```python
from build123d import *

# Parameters (mm, degrees)
BOSS_EXTRUDE1_DEPTH = 20
SKETCH2_R           = 3.7
CUT_EXTRUDE1_DEPTH  = 20
SKETCH3_R           = 3.7
CUT_EXTRUDE2_DEPTH  = 20


with BuildPart() as part:
    # Sketch1 → Boss-Extrude1 (new body)
    with BuildSketch(Plane.XY):
        Polygon((1.5, -10), (18.5, -10), (18.5, -7), (1.5, -7), (1.5, 10), (-1.5, 10), (-1.5, -10), align=None)
    extrude(amount=BOSS_EXTRUDE1_DEPTH)

    # Sketch2 → Cut-Extrude1 (cut)
    with BuildSketch(Plane(origin=(0, -7, 0), x_dir=(1, 0, 0), z_dir=(0, 1, 0))):
        with Locations(Location((10, -10, 0), (0, 0, 270))):
            Circle(SKETCH2_R)
    extrude(amount=-CUT_EXTRUDE1_DEPTH, mode=Mode.SUBTRACT)

    # Sketch3 → Cut-Extrude2 (cut)
    with BuildSketch(Plane(origin=(1.5, 0, 0), x_dir=(0, 0, -1), z_dir=(1, 0, 0))):
        with Locations(Location((-10, 0, 0), (0, 0, 90))):
            Circle(SKETCH3_R)
    extrude(amount=-CUT_EXTRUDE2_DEPTH, mode=Mode.SUBTRACT)


solid = part.part
```
The model under review builds one solid part; all positions refer to its coordinate system, in mm. A direction names the side the tool comes from. Round coordinates to 2 decimals unless told otherwise and drop trailing zeros. Write each loop counter-clockwise with the first axis right and the second up, starting at its lowest first coordinate (ties: lowest second). Pieces come first, ordered by that corner, then holes. Notation, with made-up numbers: (53.25, 32) - (82.25, 32) arc R20 cw to (82.25, 62) - close; hole circle Ø6 at (86, -38.5). An arc over 180 degrees is marked (long way). Answer as CSV lines item,"result". Start each with the question number.
(1) Draft analysis for pull direction Y (two halves, no side actions). For faces 3 (the flat face through (0, 10, 10)), 4 (the flat face through (6, -10, 10)), 5 (the cylindrical face through (0.02, -0.48, 13.67)), state which applies: pulls with the +Y half, pulls with the -Y half, needs draft (parallel to the pull), parting line crosses it, or undercut.
(2) We need section D-D on y = -8. State the section outline as (x, z) points, plus the area to 3 significant figures.
(3) To check wall thickness, follow line 1 (Z direction, x = 0.5, y = 0); line 2 (X direction, y = -8.25, z = 10); line 3 (Y direction, x = 8.5, z = 2.5). State the ranges of each line that lie inside material, in increasing order.
(4) We need section B-B on z = 13. State the section outline as (x, y) points, plus the area to 3 significant figures.
(5) For pin 1 Ø4.5 at (y, z) = (0, 10) entering from -X; pin 2 Ø6 at (x, z) = (5.5, 3.5) entering from +Y; pin 3 Ø4 at (y, z) = (0, 3.5) entering from +X, all flat-tipped, find the tip position at first contact; note any pin that passes through.
(6) We need section A-A on y = 0. State the section outline as (x, z) points, plus the area to 3 significant figures.
(7) We need section C-C on x = 10. State the section outline as (y, z) points, plus the area to 3 significant figures.
(8) For faces 1 (the flat face through (14, -7, 10)), 2 (the flat face through (1, -4, 20)), list the 3-axis set-ups (+Z, -Z, +X, -X, +Y, -Y) from which the entire face can be reached by the end or side of a thin tool; tool diameter is ignored.
Worked answers:
1,face 3,"pulls with the +Y half"
1,face 4,"pulls with the -Y half"
1,face 5,"undercut"
2,outline,"(-1.5, 0) - (18.5, 0) - (18.5, 20) - (-1.5, 20) - close; hole circle Ø7.4 at (10, 10)"
2,area,"357 mm²"
3,line 1,"0 to 6.3, 13.7 to 20"
3,line 2,"-1.5 to 6.3, 13.7 to 18.5"
3,line 3,"-10 to -7"
4,outline,"(-1.5, -10) - (7.83, -10) - (7.83, -7) - (1.5, -7) - (1.5, -2.17) - (-1.5, -2.17) - close; (-1.5, 2.17) - (1.5, 2.17) - (1.5, 10) - (-1.5, 10) - close; (12.17, -10) - (18.5, -10) - (18.5, -7) - (12.17, -7) - close"
4,area,"85.0 mm²"
5,pin 1,"through"
5,pin 2,"y = -7"
5,pin 3,"x = 1.5"
6,outline,"(-1.5, 0) - (1.5, 0) - (1.5, 6.3) - (-1.5, 6.3) - close; (-1.5, 13.7) - (1.5, 13.7) - (1.5, 20) - (-1.5, 20) - close"
6,area,"37.8 mm²"
7,outline,"(-10, 0) - (-7, 0) - (-7, 6.3) - (-10, 6.3) - close; (-10, 13.7) - (-7, 13.7) - (-7, 20) - (-10, 20) - close"
7,area,"37.8 mm²"
8,face 1,"+Z, -Z, +X, +Y"
8,face 2,"+Z, +X, -X, +Y, -Y"
